Build history of the part. All positions in model axes, mm. A direction names the side the tool comes from. Give positions to 0.01 mm unless a question says otherwise; leave off trailing zeros. Order: outer loops, then holes, each group sorted by start corner. A loop starts at its lowest first (then second) coordinate and runs counter-clockwise, first axis right, second up. Notation, with made-up numbers: (-12, -22.75) -> (0, -22.75) arc R6 ccw to (0, -11.75) -> close; hole circle Ø5 at (18.25, 31.25). An arc over 180 degrees is marked (long way). One line per item, written item: value. Start each with the question number.
(1) Saw through at A-A on y = -49. Give the cut face in (x, z).
(2) Two-plate mould, pull along Y, no slides. Class faces 6 (the flat face through (-77, -34.687, -2)), 7 (the flat face through (-78, -84.187, -2)), 8 (the flat face through (-77, -80.187, -3)): +Y half, -Y half, draft (parallel to the pull), parting line (faces both ways), or undercut.
(3) Probe line 1 (Y direction, x = -86.5, z = -4); line 2 (X direction, y = -57.5, z = -0.75); line 3 (Z direction, x = -95, y = -49.5). List the from-to ranges inside material, lowest first.
(4) Saw through at B-B on x = -83. Give the cut face in (y, z).
(5) Which spindle directions (+Z, -Z, +X, -X, +Y, -Y) get a long thin tool onto all of the face, cutting with end or side? Do faces 1 (the flat face through (-77, -59, 3)), 2 (the flat face through (-54, -52.702, -4)), 3 (the cylindrical face through (-99.99, -72.16, -2.47)), 4 (the flat face through (-56.518, -59, -3)), 5 (the cylindrical face through (-54.49, -69.226, -2.208)). Say none if no direction does.
(6) Pin check, flat tips, straight feed: pin 1 (3 mm diameter, centred on x = -73.5, y = -69, fed in from -Z); pin 2 (5 mm diameter, centred on y = -67.128, z = -2.3, fed in from +X); pin 3 (2 mm diameter, centred on x = -55.5, z = -3, fed in from -Y); pin 4 (3 mm diameter, centred on x = -53.5, z = -3.5, fed in from +Y). Stop position of each tip, or through.
(7) Saw through at C-C on z = 1. Give the cut face in (x, y) (3 decimals).
(8) Saw through at D-D on z = -2.3. Count the separate pieces of the cut face and the enclosed holes in it, plus the area to 3 significant figures.
```python
from build123d import *

# Parameters (mm, degrees)
EXTRUDE_1_DEPTH     = 3
EXTRUDE_START       = -6
EXTRUDE_2_DEPTH     = 6
SKETCH_2_R          = 2.1
CUT_EXTRUDE_1_DEPTH = 4
SKETCH_3_R          = 2.1
CUT_EXTRUDE_2_DEPTH = 4
M2_5X0_45_1_D       = 2.05
SKETCH_8_W          = 9.616
SKETCH_8_H          = 8.8
CUT_EXTRUDE_3_DEPTH = 4.4
M2_5X0_45_2_D       = 2.05


with BuildPart() as part:
    # 草图1 → 凸台-拉伸1 (new body)
    with BuildSketch(Plane.XY):
        with BuildLine():
            Line((-95.018, -34.687), (-59.518, -34.687))
            ThreePointArc((-59.518, -34.687), (-54.568252532, -36.737252532), (-52.518, -41.687))
            Line((-52.518, -41.687), (-52.518, -77.187))
            ThreePointArc((-52.518, -77.187), (-54.568252532, -82.136747468), (-59.518, -84.187))
            Line((-59.518, -84.187), (-95.018, -84.187))
            ThreePointArc((-95.018, -84.187), (-99.967747468, -82.136747468), (-102.018, -77.187))
            Line((-102.018, -77.187), (-102.018, -41.687))
            ThreePointArc((-102.018, -41.687), (-99.967747468, -36.737252532), (-95.018, -34.687))
        make_face()
    extrude(amount=EXTRUDE_1_DEPTH)

    # 草图1<3> → 凸台-拉伸2 (add)
    with BuildSketch(Plane.XY.offset(EXTRUDE_START)):
        with BuildLine():
            Line((-59.518, -34.687), (-95.018, -34.687))
            ThreePointArc((-95.018, -34.687), (-99.967747468, -36.737252532), (-102.018, -41.687))
            Line((-102.018, -41.687), (-102.018, -77.187))
            ThreePointArc((-102.018, -77.187), (-99.967747468, -82.136747468), (-95.018, -84.187))
            Line((-95.018, -84.187), (-59.518, -84.187))
            ThreePointArc((-59.518, -84.187), (-54.568252532, -82.136747468), (-52.518, -77.187))
            Line((-52.518, -77.187), (-52.518, -41.687))
            ThreePointArc((-52.518, -41.687), (-54.568252532, -36.737252532), (-59.518, -34.687))
        make_face()
        with BuildLine():
            Line((-61.517999092, -80.187), (-94.518000908, -80.187))
            Line((-94.518000908, -80.187), (-95.018, -80.187))
            ThreePointArc((-95.018, -80.187), (-97.139320344, -79.308320344), (-98.018, -77.187))
            Line((-98.018, -77.187), (-98.018, -41.687))
            ThreePointArc((-98.018, -41.687), (-97.139320344, -39.565679656), (-95.018, -38.687))
            Line((-95.018, -38.687), (-59.518, -38.687))
            ThreePointArc((-59.518, -38.687), (-57.396679656, -39.565679656), (-56.518, -41.687))
            Line((-56.518, -41.687), (-56.518, -77.187))
            ThreePointArc((-56.518, -77.187), (-57.396679656, -79.308320344), (-59.518, -80.187))
            Line((-59.518, -80.187), (-61.517999092, -80.187))
        make_face(mode=Mode.SUBTRACT)
    extrude(amount=EXTRUDE_2_DEPTH)

    # 草图2 → 切除-拉伸1 (cut)
    with BuildSketch(Plane.ZY.offset(102.018)):
        with Locations((-2.6, -67.128)):
            Circle(SKETCH_2_R)
    extrude(amount=-CUT_EXTRUDE_1_DEPTH, mode=Mode.SUBTRACT)

    # 草图3 → 切除-拉伸2 (cut)
    with BuildSketch(Plane(origin=(-52.518, 0, 0), x_dir=(0, 0, -1), z_dir=(1, 0, 0))):
        with Locations(Location((2.3, -67.128, 0), (0, 0, 90))):
            Circle(SKETCH_3_R)
    extrude(amount=-CUT_EXTRUDE_2_DEPTH, mode=Mode.SUBTRACT)

    # M2.5x0.45 螺纹孔1 (through all)
    with Locations(Plane.ZY.offset(102.018)):
        with Locations((-2.6, -61.078), (-2.6, -73.178)):
            Hole(M2_5X0_45_1_D / 2)

    # 草图8 → 切除-拉伸3 (cut)
    with BuildSketch(Plane(origin=(0, 0, -6), x_dir=(-1, 0, 0), z_dir=(0, 0, -1))):
        with Locations((57.326, -48.302)):
            Rectangle(SKETCH_8_W, SKETCH_8_H)
    extrude(amount=-CUT_EXTRUDE_3_DEPTH, mode=Mode.SUBTRACT)

    # M2.5x0.45 螺纹孔2 (through all)
    with Locations(Plane.XY.offset(3)):
        with Locations((-89.018, -44.497), (-69.018, -44.497), (-69.018, -75.497), (-89.018, -75.497)):
            Hole(M2_5X0_45_2_D / 2)


solid = part.part
```
Results below:
1. outline: (-102.02, -6) -> (-98.02, -6) -> (-98.02, 0) -> (-56.52, 0) -> (-56.52, -1.6) -> (-52.52, -1.6) -> (-52.52, 3) -> (-102.02, 3) -> close
2. face 6: +Y half
2. face 7: -Y half
2. face 8: undercut
3. line 1: y = -84.19 to -80.19, -38.69 to -34.69
3. line 2: x = -102.02 to -98.02, -56.52 to -52.52
3. line 3: z = 0 to 3
4. outline: (-84.19, -6) -> (-80.19, -6) -> (-80.19, 0) -> (-38.69, 0) -> (-38.69, -6) -> (-34.69, -6) -> (-34.69, 3) -> (-84.19, 3) -> close
5. face 1: +Z, +X, -X, +Y, -Y
5. face 2: -Z, +X
5. face 3: +X, -X
5. face 4: -Z
5. face 5: +X
6. pin 1: stops at z = 0
6. pin 2: stops at x = -52.52
6. pin 3: stops at y = -83.5
6. pin 4: stops at y = -36.34
7. outline: (-102.018, -77.187) arc R7 ccw to (-95.018, -84.187) -> (-59.518, -84.187) arc R7 ccw to (-52.518, -77.187) -> (-52.518, -41.687) arc R7 ccw to (-59.518, -34.687) -> (-95.018, -34.687) arc R7 ccw to (-102.018, -41.687) -> close; hole circle Ø2.05 at (-89.018, -75.497); hole circle Ø2.05 at (-89.018, -44.497); hole circle Ø2.05 at (-69.018, -75.497); hole circle Ø2.05 at (-69.018, -44.497)
8. separate pieces: 7
8. enclosed holes: 0
8. area: 594 mm²
